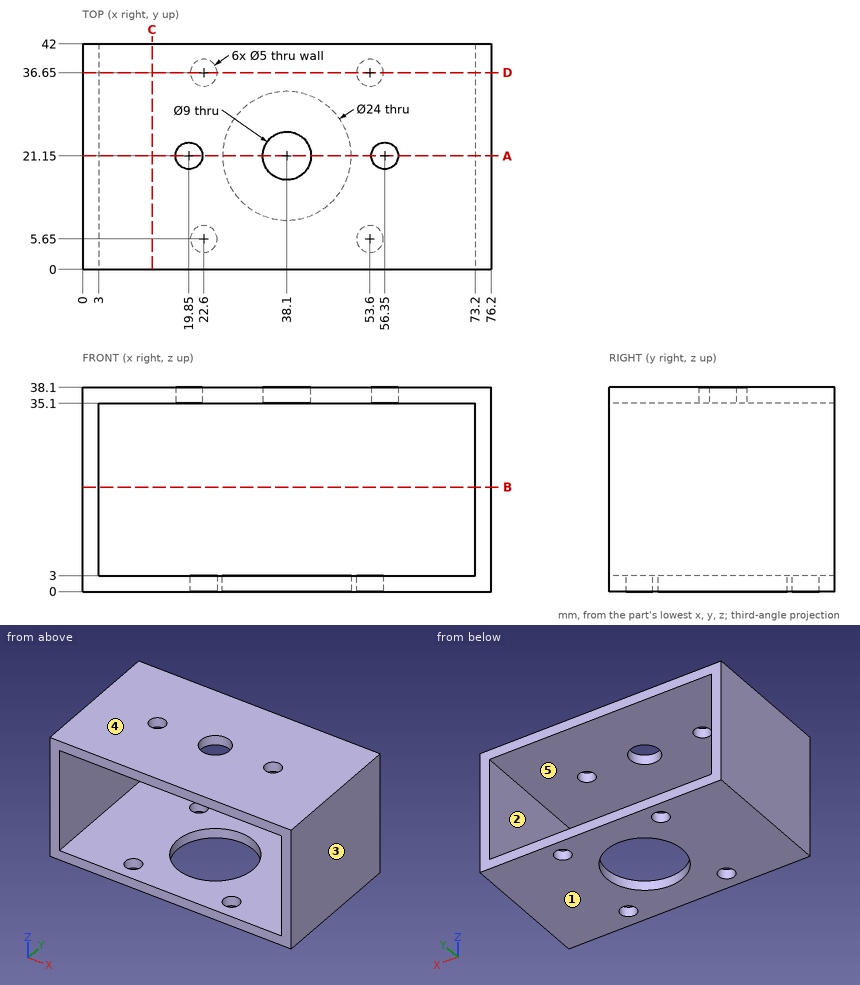
Source: three-view drawing plus pictorial views. Frame: mm from the lowest corner of the part. A direction names the side the tool comes from. Give positions to 0.01 mm unless a question says otherwise; leave off trailing zeros. Order: outer loops, then holes, each group sorted by start corner. A loop starts at its lowest first (then second) coordinate and runs counter-clockwise, first axis right, second up.
1. Section C-C on x = 13. Return the cut outline in (y, z), and give its area (3 significant figures).
Derived:
outline: (0, 0) - (42, 0) - (42, 3) - (0, 3) - close; (0, 35.1) - (42, 35.1) - (42, 38.1) - (0, 38.1) - close
area: 252 mm2
2. Section B-B on z = 19.5. Return the cut outline in (x, y).
Derived:
outline: (0, 0) - (3, 0) - (3, 42) - (0, 42) - close; (73.2, 0) - (76.2, 0) - (76.2, 42) - (73.2, 42) - close
3. Reachability of the marked faces 4 and 5 from +Z, -Z, +X, -X, +Y, -Y: full face, straight path, thin tool, end or side. Return the list, or none.
Derived:
face 4: +Z, +X, -X, +Y, -Y
face 5: +Y, -Y
4. Section A-A on y = 21.15. Return the cut outline in (x, z), and give its area (3 significant figures).
Derived:
outline: (0, 0) - (26.1, 0) - (26.1, 3) - (3, 3) - (3, 35.1) - (17.35, 35.1) - (17.35, 38.1) - (0, 38.1) - close; (22.35, 35.1) - (33.6, 35.1) - (33.6, 38.1) - (22.35, 38.1) - close; (42.6, 35.1) - (53.85, 35.1) - (53.85, 38.1) - (42.6, 38.1) - close; (50.1, 0) - (76.2, 0) - (76.2, 38.1) - (58.85, 38.1) - (58.85, 35.1) - (73.2, 35.1) - (73.2, 3) - (50.1, 3) - close
area: 521 mm2
5. Section D-D on y = 36.65. Return the cut outline in (x, z).
Derived:
outline: (0, 0) - (20.1, 0) - (20.1, 3) - (3, 3) - (3, 35.1) - (73.2, 35.1) - (73.2, 3) - (56.1, 3) - (56.1, 0) - (76.2, 0) - (76.2, 38.1) - (0, 38.1) - close; (25.1, 0) - (51.1, 0) - (51.1, 3) - (25.1, 3) - close
6. Pin query (flat end, axial travel): pin 1 (4 mm diameter, centred on x = 56.35, y = 21.15, fed in from +Z); pin 2 (3 mm diameter, centred on x = 22.6, y = 36.65, fed in from -Z). Return the tip coordinate at first contact, or that it passes through.
Derived:
pin 1: stops at z = 3
pin 2: stops at z = 35.1
7. Mould query, pull axis X, two halves, no side actions, for the marked faces 1, 2 and 3. Classes: released by +X, released by -X, zero draft, split by the parting line, or undercut.
Derived:
face 1: zero draft
face 2: undercut
face 3: released by +X
8. Material intervals for L1, parallel to Y at x = 53.6, z = 1.75; L2, parallel to X at y = 21, z = 37; L3, parallel to X at y = 5, z = 6.5, sorted ascending.
Derived:
L1: y = 0 to 3.15, 8.15 to 34.15, 39.15 to 42
L2: x = 0 to 17.35, 22.35 to 33.6, 42.6 to 53.85, 58.85 to 76.2
L3: x = 0 to 3, 73.2 to 76.2
